Model file for the job. Use its own axes, mm. A direction names the side the tool comes from. Round coordinates to 2 decimals unless told otherwise and drop trailing zeros. Write each loop counter-clockwise with the first axis right and the second up, starting at its lowest first coordinate (ties: lowest second). Pieces come first, ordered by that corner, then holes.
```python
from build123d import *

# Parameters (mm, degrees)
ESQUISSE1_W             = 70
ESQUISSE1_H             = 40
BOSS_EXTRU_1_DEPTH      = 3
BOSS_EXTRU_2_DEPTH      = 3
ESQUISSE3_W             = 70
ESQUISSE3_H             = 30
ENL_V_MAT_EXTRU_1_DEPTH = 3
CONG_1_R                = 10
CONG_2_R                = 5


with BuildPart() as part:
    # Esquisse1 → Boss.-Extru.1 (new body)
    with BuildSketch(Plane.XY):
        Rectangle(ESQUISSE1_W, ESQUISSE1_H)
    extrude(amount=BOSS_EXTRU_1_DEPTH)

    # Esquisse2 → Boss.-Extru.2 (add)
    with BuildSketch(Plane(origin=(35, 0, 0), x_dir=(0, 0, -1), z_dir=(1, 0, 0))):
        with BuildLine():
            Line((-14.5, 20), (-20.5, 20))
            Line((-20.5, 20), (-39.5, -20))
            Line((-39.5, -20), (-36.086461528, -20))
            Line((-36.086461528, -20), (-7.955603951, -20))
            Line((-7.955603951, -20), (4.955603951, -20))
            Line((4.955603951, -20), (33.086461528, -20))
            Line((33.086461528, -20), (36.5, -20))
            Line((36.5, -20), (17.5, 20))
            Line((17.5, 20), (11.5, 20))
            ThreePointArc((11.5, 20), (7.692388155, 10.807611845), (-1.5, 7))
            ThreePointArc((-1.5, 7), (-10.692388155, 10.807611845), (-14.5, 20))
        make_face()
    boss_extru_2 = extrude(amount=BOSS_EXTRU_2_DEPTH)

    # Symétrie1: Boss.-Extru.2 across plane
    add(boss_extru_2.mirror(Plane(origin=(0, 0, 0), x_dir=(0, 0, 1), z_dir=(1, 0, 0))))

    # Esquisse3 → Enlèv. mat.-Extru.1 (cut)
    with BuildSketch(Plane.XY.offset(3)):
        with Locations((0, 5)):
            Rectangle(ESQUISSE3_W, ESQUISSE3_H)
    extrude(amount=-ENL_V_MAT_EXTRU_1_DEPTH, mode=Mode.SUBTRACT)

    # Congé1
    cong_1_edges = [part.edges().sort_by_distance(p)[0] for p in [
        (-35, -10, 1.5),
        (35, -10, 1.5),
    ]]
    fillet(cong_1_edges, radius=CONG_1_R)

    # Congé2
    cong_2_edges = [part.edges().sort_by_distance(p)[0] for p in [
        (35, -5, 0),
        (-35, -5, 0),
        (-35, -5, 3),
        (35, -5, 3),
    ]]
    fillet(cong_2_edges, radius=CONG_2_R)


solid = part.part
```
1) Pull direction X, two halves, no side cores. Call faces 5 (the face through (38, -4, 2)), 6 (the face through (-36, 20, -15)), 7 (the face through (33, -6, 1)), 8 (the face through (0, -16, 3)): released by +X, released by -X, zero draft, split by the parting line, or undercut.
2) Wall check: probe 1 along X at (y, z) = (-15.5, 15.5); probe 2 along Z at (x, y) = (-16.5, -13); probe 3 along Y at (x, z) = (-17, 1). Give the ranges that are in metal, low to high.
3) Cut at C-C on y = -7.5. List the corners of the cut face in (x, z).
4) Which spindle directions (+Z, -Z, +X, -X, +Y, -Y) get a long thin tool onto all of the face, cutting with end or side? Do faces 1 (the face through (-38, -4, 2)), 2 (the face through (-33, -12, 4)), 3 (the face through (-33, -6, 1)), 4 (the face through (34, -12, -2)). Say none if no direction does.
5) Cut at D-D on x = -3.5. List the corners of the cut face in (y, z), and give its area (3 significant figures).
6) Flat gauge pins, fed straight in: pin 1 Ø12.5 at (x, y) = (2, -15.5) entering from -Z; pin 2 Ø5.5 at (x, y) = (8, -12.5) entering from +Z; pin 3 Ø1 at (x, z) = (-24, 5) entering from -Y; pin 4 Ø0.9 at (x, z) = (5, 1.5) entering from +Y. Where does each tip first touch, or does it go through?
7) Cut at B-B on z = -23.5. List the corners of the cut face in (x, y).
8) Cut at A-A on y = 16. List the corners of the cut face in (x, z).
Result sheet:
1. face 5: released by +X
1. face 6: zero draft
1. face 7: undercut
1. face 8: undercut
2. probe 1: x = -38 to -35, 35 to 38
2. probe 2: z = 0 to 3
2. probe 3: y = -20 to -10
3. outline: (-38, -30.56) - (-35, -30.56) - (-35, -5) arc R5 cw to (-31.61, -0.27) - (-31.61, 3.27) arc R5 cw to (-35, 8) - (-35, 33.56) - (-38, 33.56) - close; (31.61, -0.27) arc R5 cw to (35, -5) - (35, -30.56) - (38, -30.56) - (38, 33.56) - (35, 33.56) - (35, 8) arc R5 cw to (31.61, 3.27) - close
4. face 1: +Z, -Z, -X, +Y, -Y
4. face 2: +Z, +Y, -Y
4. face 3: +Z, -Z, +Y
4. face 4: -Z, +Y, -Y
5. outline: (-20, 0) - (-10, 0) - (-10, 3) - (-20, 3) - close
5. area: 30.0 mm2
6. pin 1: stops at z = 0
6. pin 2: stops at z = 3
6. pin 3: passes through
6. pin 4: stops at y = -10
7. outline: (-38, -20) - (-35, -20) - (-35, 7.37) - (-38, 7.37) - close; (35, -20) - (38, -20) - (38, 7.37) - (35, 7.37) - close
8. outline: (-38, -19.4) - (-35, -19.4) - (-35, -10.87) - (-38, -10.87) - close; (-38, 13.87) - (-35, 13.87) - (-35, 22.4) - (-38, 22.4) - close; (35, -19.4) - (38, -19.4) - (38, -10.87) - (35, -10.87) - close; (35, 13.87) - (38, 13.87) - (38, 22.4) - (35, 22.4) - close
